Could you check a few things on this model? Use its own coordinates, in mm. A direction names the side the tool comes from. Coordinates: 2 decimals unless noted, no trailing zeros. Loops run counter-clockwise (first coordinate to the right, second up) from the corner with the lowest first, then second, coordinate; pieces in that order, holes last. Notation, with made-up numbers: (-33, -15) - (4, -15) arc R12 ccw to (4, 4) - close; hole circle Ø9 at (86, 4). An arc over 180 degrees is marked (long way). One line per item, written item: value. Start each with the question number.
(1) On a 3-axis mill with a long thin cutter (end or side, diameter ignored), from which of +Z, -Z, +X, -X, +Y, -Y can I reach the whole of each face in a straight line? I mean faces 4 (the face through (6, -3, 7.6)), 5 (the face through (-1, -5, 3)), 6 (the face through (5.589, -2.317, 6.121)). Say none if no direction works.
(2) If we section it at A-A on x = 0: Write out the boundary of the cut face in (y, z), then the cut area to 3 significant figures.
(3) I'm going to push flat-ended pins straight in: P1, Ø6, axis at x = 0, y = -2, coming from the -Z side; P2, Ø4, axis at y = -9.5, z = 5, coming from the +X side; P3, Ø13.5, axis at x = 2.5, y = 2, coming from the +Z side; P4, Ø1, axis at y = -5, z = 4.5, coming from the +X side. Where does each tip first touch, or does it pass through?
(4) If we section it at D-D on z = 2.25: Write out the boundary of the cut face in (x, y).
(5) If we section it at C-C on z = 5.5: Write out the boundary of the cut face in (x, y).
(6) If we mould it in two halves opening along X, with no side actions, what happens to faces 1 (the face through (6, 2, 0)), 2 (the face through (-1.062, -4.783, 3.811)), 3 (the face through (-8.06, -12.65, 3.79))? For each: pulls with the +X half, pulls with the -X half, needs draft (parallel to the pull), parting line crosses it, or undercut.
(7) If I drill on line 1 along Y through (x, z) = (0, 3.95); line 2 along X through (y, z) = (0.75, 2); line 3 along Y through (x, z) = (0, 1.15), over which ranges is the centre line in solid material (lowest first)? Write a range as from..to.
```python
from build123d import *

# Parameters (mm, degrees)
SKETCH_1_R          = 15
EXTRUDE_1_DEPTH     = 7.6
SKETCH_2_R          = 6.05
CUT_EXTRUDE_1_DEPTH = 3
SKETCH_3_R          = 6
CUT_EXTRUDE_2_DEPTH = 3
SKETCH_4_R          = 4.9
CUT_EXTRUDE_3_DEPTH = 22.706220307
FILLET_1_R          = 3


with BuildPart() as part:
    # 草图1 → 凸台-拉伸1 (new body)
    with BuildSketch(Plane.XY):
        with Locations(Location((0, 0, 0), (0, 0, 180))):
            Circle(SKETCH_1_R)
    extrude(amount=EXTRUDE_1_DEPTH)

    # 草图2 → 切除-拉伸1 (cut)
    with BuildSketch(Plane.XY.offset(7.6)):
        Circle(SKETCH_2_R)
    extrude(amount=-CUT_EXTRUDE_1_DEPTH, mode=Mode.SUBTRACT)

    # 草图3 → 切除-拉伸2 (cut)
    with BuildSketch(Plane(origin=(0, 0, 0), x_dir=(-1, 0, 0), z_dir=(0, 0, -1))):
        Circle(SKETCH_3_R)
    extrude(amount=-CUT_EXTRUDE_2_DEPTH, mode=Mode.SUBTRACT)

    # 草图4 → 切除-拉伸3 (cut, through all)
    with BuildSketch(Plane.XY.offset(4.6)):
        Circle(SKETCH_4_R)
    extrude(amount=-CUT_EXTRUDE_3_DEPTH, mode=Mode.SUBTRACT)

    # 圆角1
    fillet_1_edges = [part.edges().sort_by_distance(p)[0] for p in [
        (15, 0, 0),
        (15, 0, 7.6),
    ]]
    fillet(fillet_1_edges, radius=FILLET_1_R)


solid = part.part
```
Values:
1. face 4: +Z, +X, -X, +Y, -Y
1. face 5: -Z
1. face 6: +Z
2. outline: (-15, 3) arc R3 ccw to (-12, 0) - (-6, 0) - (-6, 3) - (-4.9, 3) - (-4.9, 4.6) - (-6.05, 4.6) - (-6.05, 7.6) - (-12, 7.6) arc R3 ccw to (-15, 4.6) - close; (4.9, 3) - (6, 3) - (6, 0) - (12, 0) arc R3 ccw to (15, 3) - (15, 4.6) arc R3 ccw to (12, 7.6) - (6.05, 7.6) - (6.05, 4.6) - (4.9, 4.6) - close
2. area: 132 mm2
3. P1: stops at z = 3
3. P2: stops at x = 12.98
3. P3: stops at z = 7.6
3. P4: stops at x = 14.31
4. outline: circle Ø29.81 at (0, 0); hole circle Ø12 at (0, 0)
5. outline: circle Ø29.72 at (0, 0); hole circle Ø12.1 at (0, 0)
6. face 1: needs draft
6. face 2: undercut
6. face 3: parting line crosses it
7. line 1: y = -15..-4.9, 4.9..15
7. line 2: x = -14.81..-5.95, 5.95..14.81
7. line 3: y = -14.36..-6, 6..14.36
